Check sheet for the drawn part. Datum: minimum x, y, z corner. Units: mm. Give positions to 0.01 mm unless a question says otherwise; leave off trailing zeros. Loops run counter-clockwise (first coordinate to the right, second up) from the corner with the lowest first, then second, coordinate; pieces in that order, holes last. Notation, with made-up numbers: (66.5, -19.75) -> (82.5, -19.75) arc R33 ccw to (82.5, 9.25) -> close; hole circle Ø6 at (12.25, 69.25). An arc over 180 degrees is marked (long way). One line per question, with ' | ' between items.
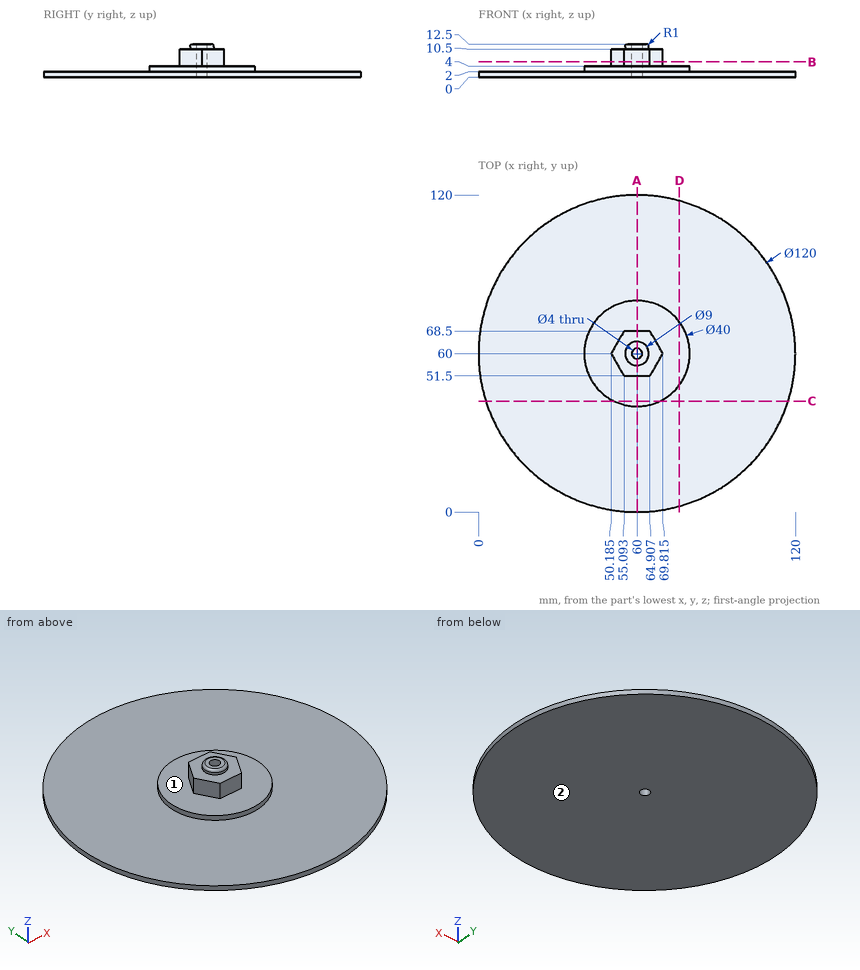
Item 1: Sectioned sample at C-C (y = 42). Record the cut outline in (x, z), plus the area to 3 significant figures.
Result:
outline: (2.76, 0) -> (117.24, 0) -> (117.24, 2) -> (68.72, 2) -> (68.72, 4) -> (51.28, 4) -> (51.28, 2) -> (2.76, 2) -> close | area: 264 mm2
Item 2: Scan lines: probe 1 along Y at (x, z) = (60, 3.5); probe 2 along Y at (x, z) = (60, 5); probe 3 along Z at (x, y) = (45.5, 80.5). Record each from-to range of solid material in increasing order.
Result:
probe 1: 40 to 58, 62 to 80 | probe 2: 51.5 to 58, 62 to 68.5 | probe 3: 0 to 2
Item 3: Depth check by flat-ended pin: pin 1 Ø3 at (x, z) = (58.5, 7) entering from -Y; pin 2 Ø8 at (x, y) = (59.5, 89.5) entering from +Z; pin 3 Ø3 at (x, z) = (61, 6) entering from +Y; pin 4 Ø3 at (x, y) = (60, 60) entering from +Z. Enter the tip coordinate at first touch or a pass-through.
Result:
pin 1: y = 51.5 | pin 2: z = 2 | pin 3: y = 68.5 | pin 4: through
Item 4: Release check for a two-part mould opening along Z. For the marked faces 1 and 2 record: pulls with the +Z half, pulls with the -Z half, needs draft (parallel to the pull), parting line crosses it, or undercut.
Result:
face 1: pulls with the +Z half | face 2: pulls with the -Z half
Item 5: Sectioned sample at D-D (x = 76). Record the cut outline in (y, z).
Result:
outline: (2.17, 0) -> (117.83, 0) -> (117.83, 2) -> (72, 2) -> (72, 4) -> (48, 4) -> (48, 2) -> (2.17, 2) -> close
Item 6: Sectioned sample at A-A (x = 60). Record the cut outline in (y, z), plus the area to 3 significant figures.
Result:
outline: (0, 0) -> (58, 0) -> (58, 12.5) -> (56.5, 12.5) arc R1 ccw to (55.5, 11.5) -> (55.5, 10.5) -> (51.5, 10.5) -> (51.5, 4) -> (40, 4) -> (40, 2) -> (0, 2) -> close; (62, 0) -> (120, 0) -> (120, 2) -> (80, 2) -> (80, 4) -> (68.5, 4) -> (68.5, 10.5) -> (64.5, 10.5) -> (64.5, 11.5) arc R1 ccw to (63.5, 12.5) -> (62, 12.5) -> close | area: 398 mm2
Item 7: Sectioned sample at B-B (z = 5.75). Record the cut outline in (x, y) (1 decimal).
Result:
outline: (50.2, 60) -> (55.1, 51.5) -> (64.9, 51.5) -> (69.8, 60) -> (64.9, 68.5) -> (55.1, 68.5) -> close; hole circle Ø4 at (60, 60)
